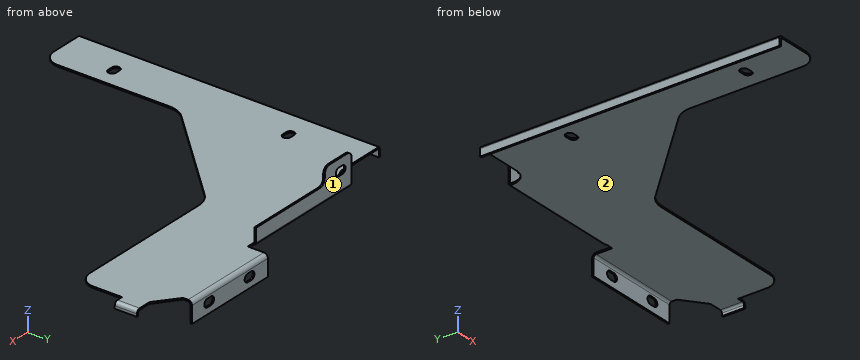
```python
from build123d import *

# Parameters (mm, degrees)
BASE_FLANGE1_DEPTH            = 1
EDGE_FLANGE1_STRIP_W          = 5
EDGE_FLANGE1_STRIP_H          = 1
EDGE_FLANGE1_STRIP_CUT_DEPTH  = 189
EDGE_FLANGE1_RELIEF_W         = 5.5
EDGE_FLANGE1_RELIEF_H         = 0.5
EDGE_FLANGE1_RELIEF_CUT_DEPTH = 1
EDGE_FLANGE1_DEPTH            = 189
CUT_EXTRUDE1_DEPTH            = 10
EDGE_FLANGE2_STRIP_W          = 7
EDGE_FLANGE2_STRIP_H          = 1
EDGE_FLANGE2_STRIP_CUT_DEPTH  = 62
EDGE_FLANGE2_RELIEF_W         = 7.5
EDGE_FLANGE2_RELIEF_H         = 0.5
EDGE_FLANGE2_RELIEF_CUT_DEPTH = 1
EDGE_FLANGE2_DEPTH            = 62
SKETCH13_W                    = 5
SKETCH13_H                    = 14
TAB1_DEPTH                    = 1
CUT_EXTRUDE4_DEPTH            = 10
EDGE_FLANGE3_STRIP_W          = 6.54
EDGE_FLANGE3_STRIP_H          = 1
EDGE_FLANGE3_STRIP_CUT_DEPTH  = 14
EDGE_FLANGE3_DEPTH            = 14
CUT_EXTRUDE3_DEPTH            = 10
EDGE_FLANGE5_DEPTH            = 78
SKETCH33_W                    = 22
SKETCH33_H                    = 10
TAB2_DEPTH                    = 1
FILLET1_R                     = 4
FILLET2_R                     = 4
CUT_EXTRUDE5_DEPTH            = 1
CUT_EXTRUDE6_DEPTH            = 1
CUT_EXTRUDE7_DEPTH            = 1


# Sheet-metal steps are written as plain solids
with BuildPart() as part:
    # Sketch1 → Base-Flange1 (new body)
    with BuildSketch(Plane.XY):
        with BuildLine():
            Line((0, 0), (0, -212.19))
            Line((0, -212.19), (20.5, -212.19))
            ThreePointArc((20.5, -212.19), (27.571067812, -209.261067812), (30.5, -202.19))
            Line((30.5, -202.19), (30.5, -131.403203436))
            ThreePointArc((30.5, -131.403203436), (31.641807012, -125.66295195), (34.893398282, -120.796601718))
            Line((34.893398282, -120.796601718), (92.574639149, -61.583398282))
            ThreePointArc((92.574639149, -61.583398282), (97.440989382, -58.331807012), (103.181240867, -57.19))
            Line((103.181240867, -57.19), (192, -57.19))
            ThreePointArc((192, -57.19), (199.071067812, -54.261067812), (202, -47.19))
            Line((202, -47.19), (202, 0))
            Line((202, 0), (0, 0))
        make_face()
    extrude(amount=-BASE_FLANGE1_DEPTH)

    # Edge-Flange1 strip (across the edge) → Edge-Flange1 strip cut (cut)
    with BuildSketch(Plane.XZ.offset(23.19)):
        with Locations((-2, -0.5)):
            Rectangle(EDGE_FLANGE1_STRIP_W, EDGE_FLANGE1_STRIP_H)
    extrude(amount=EDGE_FLANGE1_STRIP_CUT_DEPTH, mode=Mode.SUBTRACT)

    # Edge-Flange1 relief (on the sheet) → Edge-Flange1 relief cut (cut)
    with BuildSketch(Plane(origin=(0.5, -23.19, 0), x_dir=(1, 0, 0), z_dir=(0, 0, 1))):
        with Locations((-2.25, 0.25)):
            Rectangle(EDGE_FLANGE1_RELIEF_W, EDGE_FLANGE1_RELIEF_H)
    extrude(amount=-EDGE_FLANGE1_RELIEF_CUT_DEPTH, mode=Mode.SUBTRACT)

    # Edge-Flange1 section (across the edge) → Edge-Flange1 (add)
    with BuildSketch(Plane.XZ.offset(23.19)):
        with BuildLine():
            Line((-1, 0.5), (-1, 5))
            Line((-1, 5), (0, 5))
            Line((0, 5), (0, 0.5))
            ThreePointArc((0, 0.5), (0.146446609, 0.146446609), (0.5, 0))
            Line((0.5, 0), (0.5, -1))
            ThreePointArc((0.5, -1), (-0.560660172, -0.560660172), (-1, 0.5))
        make_face()
    extrude(amount=EDGE_FLANGE1_DEPTH)

    # Sketch9 → Cut-Extrude1 (cut)
    with BuildSketch(Plane.XY):
        with BuildLine():
            Line((-1, -23.19), (29, -23.19))
            ThreePointArc((29, -23.19), (36.071067812, -20.261067812), (39, -13.19))
            Line((39, -13.19), (39, 0))
            Line((39, 0), (-1, 0))
            Line((-1, 0), (-1, -23.19))
        make_face()
    extrude(amount=-CUT_EXTRUDE1_DEPTH, mode=Mode.SUBTRACT)

    # Edge-Flange2 strip (across the edge) → Edge-Flange2 strip cut (cut)
    with BuildSketch(Plane(origin=(184, 0, 0), x_dir=(0, -1, 0), z_dir=(-1, 0, 0))):
        with Locations((-2, -0.5)):
            Rectangle(EDGE_FLANGE2_STRIP_W, EDGE_FLANGE2_STRIP_H)
    extrude(amount=EDGE_FLANGE2_STRIP_CUT_DEPTH, mode=Mode.SUBTRACT)

    # Edge-Flange2 relief (on the sheet) → Edge-Flange2 relief cut (cut)
    with BuildSketch(Plane(origin=(184, -1.5, 0), x_dir=(0, -1, 0), z_dir=(0, 0, 1))):
        with Locations((-3.25, 0.25)):
            Rectangle(EDGE_FLANGE2_RELIEF_W, EDGE_FLANGE2_RELIEF_H)
        with Locations((-3.25, -62.25)):
            Rectangle(EDGE_FLANGE2_RELIEF_W, EDGE_FLANGE2_RELIEF_H)
    extrude(amount=-EDGE_FLANGE2_RELIEF_CUT_DEPTH, mode=Mode.SUBTRACT)

    # Edge-Flange2 section (across the edge) → Edge-Flange2 (add)
    with BuildSketch(Plane(origin=(184, 0, 0), x_dir=(0, -1, 0), z_dir=(-1, 0, 0))):
        with BuildLine():
            Line((-1, 1.5), (-1, 12))
            Line((-1, 12), (0, 12))
            Line((0, 12), (0, 1.5))
            ThreePointArc((0, 1.5), (0.439339828, 0.439339828), (1.5, 0))
            Line((1.5, 0), (1.5, -1))
            ThreePointArc((1.5, -1), (-0.267766953, -0.267766953), (-1, 1.5))
        make_face()
    extrude(amount=EDGE_FLANGE2_DEPTH)

    # Sketch13 → Tab1 (add)
    with BuildSketch(Plane.XY):
        with Locations((204.5, -22.19)):
            Rectangle(SKETCH13_W, SKETCH13_H)
    extrude(amount=-TAB1_DEPTH)

    # Sketch16 → Cut-Extrude4 (cut)
    with BuildSketch(Plane.XY):
        with BuildLine():
            Line((202, -15.19), (198.18765136, -15.19))
            ThreePointArc((198.18765136, -15.19), (197.864812853, -15.136454066), (197.576547726, -14.981550598))
            Line((197.576547726, -14.981550598), (184.019444818, -4.515012052))
            ThreePointArc((184.019444818, -4.515012052), (184.005123731, -4.497482662), (184, -4.475434523))
            Line((184, -4.475434523), (184, -1.5))
            Line((184, -1.5), (184, 0))
            Line((184, 0), (202, 0))
            Line((202, 0), (202, -15.19))
        make_face()
    extrude(amount=-CUT_EXTRUDE4_DEPTH, mode=Mode.SUBTRACT)

    # Edge-Flange3 strip (across the edge) → Edge-Flange3 strip cut (cut)
    with BuildSketch(Plane(origin=(207, -29.19, 0), x_dir=(-1, 0, 0), z_dir=(0, 1, 0))):
        with Locations((-2, -0.5)):
            Rectangle(EDGE_FLANGE3_STRIP_W, EDGE_FLANGE3_STRIP_H)
    extrude(amount=EDGE_FLANGE3_STRIP_CUT_DEPTH, mode=Mode.SUBTRACT)

    # Edge-Flange3 section (across the edge) → Edge-Flange3 (add)
    with BuildSketch(Plane(origin=(207, -29.19, 0), x_dir=(-1, 0, 0), z_dir=(0, 1, 0))):
        with BuildLine():
            Line((-1, 1.27), (-1, 3))
            Line((-1, 3), (0, 3))
            Line((0, 3), (0, 1.27))
            ThreePointArc((0, 1.27), (0.371974388, 0.371974388), (1.27, 0))
            Line((1.27, 0), (1.27, -1))
            ThreePointArc((1.27, -1), (-0.335132393, -0.335132393), (-1, 1.27))
        make_face()
    extrude(amount=EDGE_FLANGE3_DEPTH)

    # Sketch20 → Cut-Extrude3 (cut)
    with BuildSketch(Plane.XY):
        Polygon((122, -0.75), (122, -11.75), (38.53901494, -11.75), (38.53901494, 0), (122, 0), align=None)
    extrude(amount=-CUT_EXTRUDE3_DEPTH, mode=Mode.SUBTRACT)

    # Edge-Flange5 section (across the edge) → Edge-Flange5 (add)
    with BuildSketch(Plane(origin=(39, -11.25, -1), x_dir=(0, -1, 0), z_dir=(1, 0, 0))):
        with BuildLine():
            Line((-1, 0.5), (-1, 9))
            Line((-1, 9), (0, 9))
            Line((0, 9), (0, 0.5))
            ThreePointArc((0, 0.5), (0.146446609, 0.146446609), (0.5, 0))
            Line((0.5, 0), (0.5, -1))
            ThreePointArc((0.5, -1), (-0.560660172, -0.560660172), (-1, 0.5))
        make_face()
    extrude(amount=EDGE_FLANGE5_DEPTH)

    # Sketch33 → Tab2 (add)
    with BuildSketch(Plane(origin=(0, -10.25, 0), x_dir=(1, 0, 0), z_dir=(0, 1, 0))):
        with Locations((50, 15)):
            Rectangle(SKETCH33_W, SKETCH33_H)
    extrude(amount=-TAB2_DEPTH)

    # Fillet1
    fillet1_edges = [part.edges().sort_by_distance(p)[0] for p in [
        (61, -10.75, -10),
    ]]
    fillet(fillet1_edges, radius=FILLET1_R)

    # Fillet2
    fillet2_edges = [part.edges().sort_by_distance(p)[0] for p in [
        (39, -10.75, -20),
        (61, -10.75, -20),
    ]]
    fillet(fillet2_edges, radius=FILLET2_R)

    # Sketch35 → Cut-Extrude5 (cut)
    with BuildSketch(Plane(origin=(0, 1, 0), x_dir=(1, 0, 0), z_dir=(0, 1, 0))):
        with BuildLine():
            Line((171.5, -8), (168.5, -8))
            ThreePointArc((168.5, -8), (166, -5.5), (168.5, -3))
            Line((168.5, -3), (171.5, -3))
            ThreePointArc((171.5, -3), (174, -5.5), (171.5, -8))
        make_face()
        with BuildLine():
            Line((138.5, -8), (135.5, -8))
            ThreePointArc((135.5, -8), (133, -5.5), (135.5, -3))
            Line((135.5, -3), (138.5, -3))
            ThreePointArc((138.5, -3), (141, -5.5), (138.5, -8))
        make_face()
    extrude(amount=-CUT_EXTRUDE5_DEPTH, mode=Mode.SUBTRACT)

    # Sketch36 → Cut-Extrude6 (cut)
    with BuildSketch(Plane.XZ.offset(11.25)):
        with BuildLine():
            Line((49.5, -15), (46.5, -15))
            ThreePointArc((46.5, -15), (44, -12.5), (46.5, -10))
            Line((46.5, -10), (49.5, -10))
            ThreePointArc((49.5, -10), (52, -12.5), (49.5, -15))
        make_face()
    extrude(amount=-CUT_EXTRUDE6_DEPTH, mode=Mode.SUBTRACT)

    # Sketch38 → Cut-Extrude7 (cut)
    with BuildSketch(Plane.XY):
        with BuildLine():
            Line((16, -174.19), (19, -174.19))
            ThreePointArc((19, -174.19), (21.5, -176.69), (19, -179.19))
            Line((19, -179.19), (16, -179.19))
            ThreePointArc((16, -179.19), (13.5, -176.69), (16, -174.19))
        make_face()
        with BuildLine():
            Line((16, -64.19), (19, -64.19))
            ThreePointArc((19, -64.19), (21.5, -66.69), (19, -69.19))
            Line((19, -69.19), (16, -69.19))
            ThreePointArc((16, -69.19), (13.5, -66.69), (16, -64.19))
        make_face()
    extrude(amount=-CUT_EXTRUDE7_DEPTH, mode=Mode.SUBTRACT)


with BuildPart() as body_2:
    # Mirror1: mirrored copy
    add(part.part.mirror(Plane.XY.offset(12)))


solid = body_2.part
```
The model under review builds one solid part; all positions refer to its coordinate system, in mm. Face numbers are marked on the shaded views. A direction names the side the tool comes from. Give positions to 0.01 mm unless a question says otherwise; leave off trailing zeros. Write each loop counter-clockwise with the first axis right and the second up, starting at its lowest first coordinate (ties: lowest second). Pieces come first, ordered by that corner, then holes.
(1) Consider section A-A, the plane x = 163. Give the boundary of the cut face in (y, z).
(2) Consider section C-C, the plane y = -66.69. Give the boundary of the cut face in (x, z), and give its area (3 significant figures).
(3) For P1, Ø0.8, axis at x = 120, z = 24.5, coming from the +Y side; P2, Ø8, axis at x = 94.5, y = -34.5, coming from the -Z side; P3, Ø0.8, axis at x = 95, y = -11, coming from the +Z side; P4, Ø10, axis at x = 82.5, z = 40, coming from the -Y side, all flat-tipped, find the tip position at first contact; note any pin that passes through.
(4) Consider section B-B, the plane y = -183. Give the boundary of the cut face in (x, z), and give its area (3 significant figures).
(5) Tool access review of the marked faces 1 and 2: name each direction out of +Z, -Z, +X, -X, +Y, -Y from which nothing blocks a thin tool from reaching the whole face with its end or side.
(6) To check wall thickness, follow L1, parallel to X at y = -79.5, z = 21; L2, parallel to Z at x = 88, y = -14.5; L3, parallel to Y at x = 147, z = 13. State the ranges of each line that lie inside material, in increasing order.
Returned:
1. outline: (-57.19, 24) - (-1.5, 24) arc R1.5 cw to (0, 22.5) - (0, 12) - (1, 12) - (1, 22.5) arc R2.5 ccw to (-1.5, 25) - (-57.19, 25) - close
2. outline: (-1, 19) - (0, 19) - (0, 23.5) arc R0.5 cw to (0.5, 24) - (13.5, 24) - (13.5, 25) - (0.5, 25) arc R1.5 ccw to (-1, 23.5) - close; (21.5, 24) - (87.6, 24) - (87.6, 25) - (21.5, 25) - close
2. area: 85.2 mm2
3. P1: stops at y = -11.75
3. P2: stops at z = 24
3. P3: stops at z = 34
3. P4: passes through
4. outline: (-1, 19) - (0, 19) - (0, 23.5) arc R0.5 cw to (0.5, 24) - (30.5, 24) - (30.5, 25) - (0.5, 25) arc R1.5 ccw to (-1, 23.5) - close
4. area: 36.1 mm2
5. face 1: +Z, -Z, +X, -X, +Y
5. face 2: -Z, -Y
6. L1: x = -1 to 0
6. L2: z = 24 to 25
6. L3: y = 0 to 1
